Here's the drawing with two shaded views (mm, measured from the low corner). I have some questions. A direction names the side the tool comes from. Round coordinates to 2 decimals unless told otherwise and drop trailing zeros. Order: outer loops, then holes, each group sorted by start corner. A loop starts at its lowest first (then second) coordinate and runs counter-clockwise, first axis right, second up.
Q1. If we section it at B-B (z = 30): Count the separate pieces of the cut face and the enclosed holes in it, plus the area to 3 significant figures.
Q2. For the marked faces 1 and 2, which set-ups out of +Z, -Z, +X, -X, +Y, -Y let a thin tool reach every point of the face, with its end or its side?
Q3. If we section it at D-D (x = 84): Please give me the cut outline in (y, z).
Q4. We'd pull the mould along Y, two halves only. Please class the marked faces 3, 4 and 5: pulls with the +Y half, pulls with the -Y half, needs draft (parallel to the pull), parting line crosses it, or undercut.
Q5. If I drill on line 1 (X direction, y = 69, z = 33.5); line 2 (Y direction, x = 20, z = 42); line 3 (Y direction, x = 96.5, z = 29), over which ranges is the centre line in solid material (lowest first)?
Q6. If we section it at C-C (y = 72): Please give me the cut outline in (x, z).
Q7. If we section it at A-A (x = 9): Please give me the cut outline in (y, z), plus the area to 3 significant figures.
Q8. Will this pin go through, and if not, where does the flat tip stop? P1, Ø15.5, axis at x = 14.5, z = 32, coming from the -Y side.
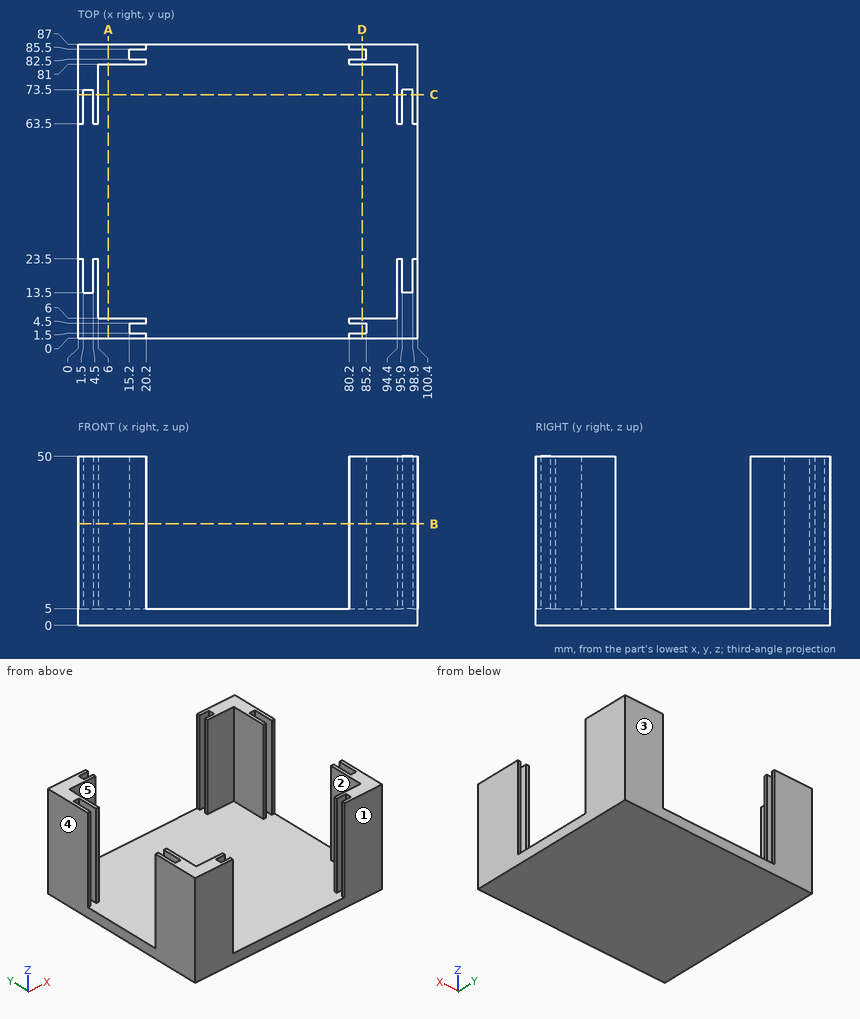
Solution:
1. separate pieces: 4
1. enclosed holes: 0
1. area: 725 mm2
2. face 1: +Z, -Z, +X, -X, -Y
2. face 2: +Z
3. outline: (0, 0) - (87, 0) - (87, 50) - (85.5, 50) - (85.5, 5) - (82.5, 5) - (82.5, 50) - (81, 50) - (81, 5) - (6, 5) - (6, 50) - (4.5, 50) - (4.5, 5) - (1.5, 5) - (1.5, 50) - (0, 50) - close
4. face 3: pulls with the +Y half
4. face 4: needs draft
4. face 5: undercut
5. line 1: x = 0 to 1.5, 4.5 to 6, 94.4 to 95.9, 98.9 to 100.4
5. line 2: y = 0 to 1.5, 4.5 to 6, 81 to 82.5, 85.5 to 87
5. line 3: y = 0 to 13.5, 73.5 to 87
6. outline: (0, 0) - (100.4, 0) - (100.4, 50) - (98.9, 50) - (98.9, 5) - (95.9, 5) - (95.9, 50) - (94.4, 50) - (94.4, 5) - (6, 5) - (6, 50) - (4.5, 50) - (4.5, 5) - (1.5, 5) - (1.5, 50) - (0, 50) - close
7. outline: (0, 0) - (87, 0) - (87, 50) - (81, 50) - (81, 5) - (6, 5) - (6, 50) - (0, 50) - close
7. area: 975 mm2
8. P1: stops at y = 0
